Model file for the job. Use its own axes, mm. Coordinates: 2 decimals unless noted, no trailing zeros. Order: outer loops, then holes, each group sorted by start corner. A loop starts at its lowest first (then second) coordinate and runs counter-clockwise, first axis right, second up. Notation, with made-up numbers: (18.25, -24) -> (55.25, -24) arc R19 cw to (55.25, 1) -> close; hole circle Ø6 at (-3, 29.5). An arc over 180 degrees is marked (long way). Write item = value, one per line. Start each with the question number.
Q1. Cut at C-C, the plane y = 1.75. List the corners of the cut face in (x, z).
Q2. Flat gauge pin, fed straight in: pin 1 (12 mm diameter, centred on x = 63, z = -138, fed in from +Y). Where does the tip first touch, or does it go through?
Q3. Cut at B-B, the plane z = -115. List the corners of the cut face in (x, y), plus the area to 3 significant figures.
Q4. Cut at D-D, the plane x = 2. List the corners of the cut face in (y, z).
Q5. Cut at A-A, the plane x = 34.5. List the corners of the cut face in (y, z).
Q6. Wall check: line 1 (X direction, y = 8.5, z = -95.5); line 2 (X direction, y = 2.75, z = -59); line 3 (Z direction, x = 54, y = 6). Give the ranges that are in metal, low to high. Write a range as from..to.
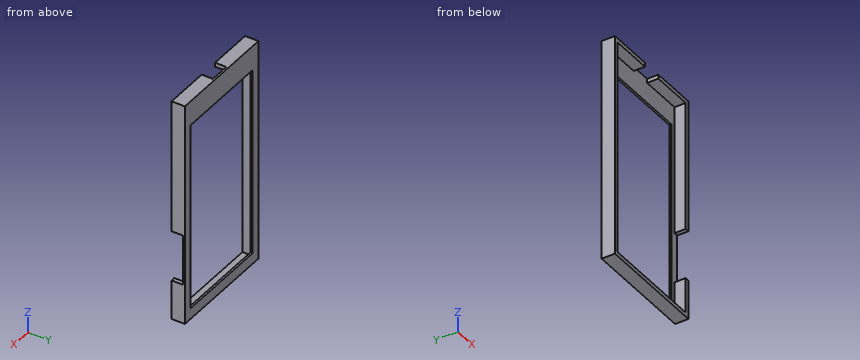
Autodesk Inventor part; units mm, degrees
ref_plane "YZ Plane" through (0, 0, 0) normal (1, 0, 0) x (0, 1, 0)
ref_plane "XZ Plane" through (0, 0, 0) normal (0, 1, 0) x (-1, 0, 0)
ref_plane "XY Plane" through (0, 0, 0) normal (0, 0, 1) x (1, 0, 0)
sketch "Sketch1" plane through (0, 0, 0) normal (0, 1, 0) x (-1, 0, 0)
  line L0 (0, 0) -> (-76.2, 0)
  line L1 (-76.2, 0) -> (-76.2, -157.8)
  line L2 (-76.2, -157.8) -> (0, -157.8)
  line L3 (0, -157.8) -> (0, 0)
  line L4 (-76.2, -157.8) -> (-79.2, -157.8)
  line L5 (-79.2, -157.8) -> (-79.2, 0)
  line L6 (-79.2, 0) -> (-76.2, 0)
  line L7 (-76.2, 0) -> (-76.2, -157.8)
  line L8 (0, -157.8) -> (3, -157.8)
  line L9 (3, -157.8) -> (3, 0)
  line L10 (3, 0) -> (0, 0)
  line L11 (0, 0) -> (0, -157.8)
  line L12 (3, 0) -> (-79.2, 0)
  line L13 (-79.2, 0) -> (-79.2, 3)
  line L14 (-79.2, 3) -> (3, 3)
  line L15 (3, 3) -> (3, 0)
  line L16 (-30.6, 0) -> (-45.6, 0)
  line L17 (-45.6, 0) -> (-45.6, 3)
  line L18 (-45.6, 3) -> (-30.6, 3)
  line L19 (-30.6, 3) -> (-30.6, 0)
  line L20 (3, -157.8) -> (-79.2, -157.8)
  line L21 (-79.2, -157.8) -> (-79.2, -160.8)
  line L22 (-79.2, -160.8) -> (3, -160.8)
  line L23 (3, -160.8) -> (3, -157.8)
  dimension "d0" = 76.2
  dimension "d1" = 157.8
  dimension "d2" = 3
  dimension "d3" = 3
  dimension "d4" = 3
  dimension "d5" = 15
  dimension "d6" = 33.6
  dimension "d7" = 33.6
  dimension "d8" = 3
extrude "Extrusion1" add sketch "Sketch1" along normal blind 8.2 contours L10 L9 L8 L3 | L0 L19 L14 L15 L10 | L8 L23 L22 L21 L4 L2 | L0 L6 L13 L14 L17 | L4 L5 L6 L1
sketch "Sketch6" plane through (0, 8.2, 0) normal (0, 1, 0) x (1, 0, 0)
  line L0 (79.2, -3) -> (79.2, 160.8)
  line L1 (-3, -3) -> (79.2, -3)
  line L2 (79.2, -3) -> (79.2, 15)
  line L3 (79.2, 15) -> (-3, 15)
  line L4 (-3, 15) -> (-3, -3)
  line L5 (-3, 160.8) -> (-3, -3)
  line L6 (-3, 160.8) -> (79.2, 160.8)
  line L7 (79.2, 160.8) -> (79.2, 152.8)
  line L8 (79.2, 152.8) -> (-3, 152.8)
  line L9 (-3, 152.8) -> (-3, 160.8)
  line L10 (-3, 15) -> (3.5, 15)
  line L11 (3.5, 15) -> (3.5, 152.8)
  line L12 (3.5, 152.8) -> (-3, 152.8)
  line L13 (-3, 152.8) -> (-3, 15)
  line L14 (79.2, 152.8) -> (72.7, 152.8)
  line L15 (72.7, 152.8) -> (72.7, 15)
  line L16 (72.7, 15) -> (79.2, 15)
  line L17 (79.2, 15) -> (79.2, 152.8)
  point P0 (0, 0)
  dimension "d22" = 18
  dimension "d23" = 8
  dimension "d24" = 6.5
  dimension "d25" = 6.5
extrude "Extrusion5" add sketch "Sketch6" along normal blind 1.5 contours L1 L4 L3 L0 | L3 L15 L8 L0 | L8 L5 L6 L0 | L5 L8 L11 L3
sketch "Sketch7" plane through (76.2, 0, -157.8) normal (-1, 0, 0) x (0, 0, 1)
  line L0 (0, 8.2) -> (157.8, 8.2)
  line L1 (0, 0) -> (157.8, 0)
  line L2 (26, 8.2) -> (63, 8.2)
  line L3 (63, 8.2) -> (63, 0)
  line L4 (63, 0) -> (26, 0)
  line L5 (26, 0) -> (26, 8.2)
  line L6 (0, 0) -> (0, 8.2)
  point P0 (26, 0)
  dimension "d28" = 37
  dimension "d29" = 26
extrude "Extrusion6" cut sketch "Sketch7" against normal blind 8 contours L0 L3 L1 L5
properties part number "caseMain"
Here are the results:
q1.outline = (-3, -160.8) -> (79.2, -160.8) -> (79.2, -131.8) -> (76.2, -131.8) -> (76.2, -157.8) -> (0, -157.8) -> (0, 0) -> (30.6, 0) -> (30.6, 3) -> (-3, 3) -> close; (45.6, 0) -> (76.2, 0) -> (76.2, -94.8) -> (79.2, -94.8) -> (79.2, 3) -> (45.6, 3) -> close
q2.pin_1 = through
q3.outline = (-3, 0) -> (0, 0) -> (0, 8.2) -> (3.5, 8.2) -> (3.5, 9.7) -> (-3, 9.7) -> close; (72.7, 8.2) -> (79.2, 8.2) -> (79.2, 9.7) -> (72.7, 9.7) -> close
q3.area = 44.1 mm²
q4.outline = (0, -160.8) -> (9.7, -160.8) -> (9.7, 3) -> (0, 3) -> (0, 0) -> (8.2, 0) -> (8.2, -157.8) -> (0, -157.8) -> close
q5.outline = (0, -160.8) -> (9.7, -160.8) -> (9.7, -152.8) -> (8.2, -152.8) -> (8.2, -157.8) -> (0, -157.8) -> close; (8.2, -15) -> (9.7, -15) -> (9.7, 3) -> (8.2, 3) -> close
q6.line_1 = -3..3.5, 72.7..79.2
q6.line_2 = -3..0, 76.2..79.2
q6.line_3 = -160.8..-157.8, 0..3
